```python
from build123d import *

# Parameters (mm, degrees)
F1_R     = 106.145751
F2_DEPTH = 25.4


with BuildPart() as f2:
    # F1 (on face) → F2 (new body)
    with BuildSketch(Plane.XZ):
        Polygon((172.641336, 115.126468), (58.517822, 83.491787), (12.095964, -25.457471), (68.332369, -129.680292), (184.879876, -150.694766), (273.975836, -72.676566), (268.529173, 45.625013), align=None)
        with Locations((148.424625, -19.180832)):
            Circle(F1_R, mode=Mode.SUBTRACT)
    extrude(amount=F2_DEPTH)


solid = f2.part
```
Input: part model. Units: mm. Frame: model coordinates. Round coordinates to 2 decimals unless told otherwise and drop trailing zeros. Loops run counter-clockwise (first coordinate to the right, second up) from the corner with the lowest first, then second, coordinate; pieces in that order, holes last. Notation, with made-up numbers: (-25.5, 72) - (-9.5, 72) arc R11 ccw to (-9.5, 79) - close; hole circle Ø7 at (69.5, 49.5). An arc over 180 degrees is marked (long way). One line per item, written item: value. Start each with the question number.
(1) Section B-B, the plane z = -121.5. Return loops of the section in (x, y).
(2) Contact query for flat-ended pins moving along their axis: P1, Ø12, axis at x = 244.5, z = 74, coming from the -Y side; P2, Ø5, axis at x = 222, y = -20.5, coming from the -Z side; P3, Ø1, axis at y = -6, z = -121, coming from the -X side; P4, Ø4, axis at x = 99.5, y = -3.5, coming from the -Z side. Output: stop coordinate, or through.
(3) Ray query, line 1 (X direction, y = -20.25, z = -42); line 2 (X direction, y = -7, z = 77); line 3 (Z direction, x = 100, y = -11.75). Return the intervals inside material, ascending. Write a range as [from, to].
(4) Section A-A, the plane x = 54. Return loops of the section in (y, z).
(5) Draft query along X for faces 1 (the flat face through (39.8, -12.5, -76.8)), 2 (the flat face through (221.256, -12.522, 79.889)), 3 (the cylindrical face through (249.67, -12.52, 12.7)), 4 (the flat face through (152.1, -25.4, -125.5)). Return one class per face: +X half, -X half, draft (parallel to the pull), parting line (faces both ways), or undercut.
(6) Section C-C, the plane y = -22. Return loops of the section in (x, z), plus the area to 3 significant figures.
Results below:
1. outline: (63.92, -25.4) - (120.18, -25.4) - (120.18, 0) - (63.92, 0) - close; (176.67, -25.4) - (218.22, -25.4) - (218.22, 0) - (176.67, 0) - close
2. P1: through
2. P2: z = -120.38
2. P3: x = 63.38
2. P4: z = -135.66
3. line 1: [21.02, 44.76], [252.09, 272.56]
3. line 2: [55.75, 103.52], [193.33, 225.24]
3. line 3: [-135.39, -113.64], [75.28, 94.99]
4. outline: (-25.4, -103.12) - (0, -103.12) - (0, -67.67) - (-25.4, -67.67) - close; (-25.4, 29.31) - (0, 29.31) - (0, 72.89) - (-25.4, 72.89) - close
5. face 1: -X half
5. face 2: +X half
5. face 3: undercut
5. face 4: draft
6. outline: (12.1, -25.46) - (68.33, -129.68) - (184.88, -150.69) - (273.98, -72.68) - (268.53, 45.63) - (172.64, 115.13) - (58.52, 83.49) - close; hole circle Ø212.29 at (148.42, -19.18)
6. area: 15,600 mm^2
